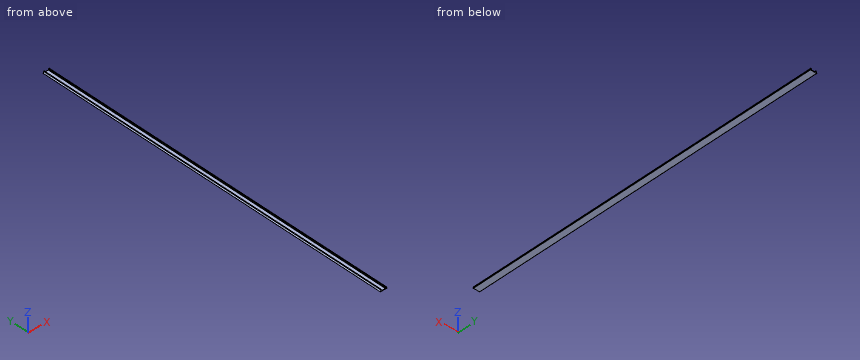
```python
from build123d import *

# Parameters (mm, degrees)
PROFILE_EXTRUDE_DEPTH = 500


with BuildPart() as part:
    # Profile Sketch → Profile Extrude (new body)
    with BuildSketch(Plane(origin=(0, 0, 0), x_dir=(1, 0, 0), z_dir=(0, 1, 0))):
        with BuildLine():
            Line((0, 0.762), (4.235793346, 0.762))
            ThreePointArc((4.235793346, 0.762), (4.559082566, 0.62808922), (4.692993346, 0.3048))
            ThreePointArc((4.692993346, 0.3048), (3.844388962, -0.212390939), (3.748927066, -1.20158399))
            ThreePointArc((3.748927066, -1.20158399), (3.415292673, -1.798270502), (2.889593346, -1.36125))
            Line((2.889593346, -1.36125), (2.889593346, -0.4572))
            ThreePointArc((2.889593346, -0.4572), (2.755682566, -0.13391078), (2.432393346, 0))
            Line((2.432393346, 0), (0, 0))
            Line((0, 0), (0, 0.762))
        make_face()
    profile_extrude = extrude(amount=PROFILE_EXTRUDE_DEPTH)

    # Profile Mirror: Profile Extrude across plane
    add(profile_extrude.mirror(Plane(origin=(0, 0, 0), x_dir=(0, 0, 1), z_dir=(1, 0, 0))))


solid = part.part
```
Source: CAD feature listing. Evaluate the final solid. Frame: model axes, mm. Give positions to 0.01 mm unless a question says otherwise; leave off trailing zeros. Order: outer loops, then holes, each group sorted by start corner. A loop starts at its lowest first (then second) coordinate and runs counter-clockwise, first axis right, second up. Notation, with made-up numbers: (35.25, 86) -> (40.25, 86) arc R20 cw to (40.25, 99) -> close; hole circle Ø6 at (20.25, -4). An arc over 180 degrees is marked (long way). Use a Markdown table: item, result.
Q1. First-contact query: P1, Ø0.7, axis at y = 144.5, z = 1, coming from the -X side; P2, Ø0.7, axis at y = 290, z = 0.5, coming from the +X side. Flat tips, straight axial feed; report the tip coordinate or a pass-through.
A:
| item | result |
|---|---|
| P1 | x = -3.78 |
| P2 | x = 3.89 |
Q2. Section B-B (x = -1). Return the cut outline in (y, z), and give its area (3 significant figures).
A:
| item | result |
|---|---|
| outline | (0, -0.76) -> (500, -0.76) -> (500, 0) -> (0, 0) -> close |
| area | 381 mm^2 |
Q3. Material intervals for line 1 (X direction, y = 278, z = 0.9); line 2 (X direction, y = 213, z = 1.5); line 3 (X direction, y = 121, z = -0.4), sorted ascending. Write a range as [from, to].
A:
| item | result |
|---|---|
| line 1 | [-3.68, -2.89], [2.89, 3.68] |
| line 2 | [-3.76, -2.91], [2.91, 3.76] |
| line 3 | [-4.68, 4.68] |
Q4. Section A-A (y = 308). Return the cut outline in (x, z), and give its area (3 significant figures).
A:
| item | result |
|---|---|
| outline | (-4.69, -0.3) arc R0.46 ccw to (-4.24, -0.76) -> (4.24, -0.76) arc R0.46 ccw to (4.69, -0.3) arc R1.11 cw to (3.75, 1.2) arc R0.44 ccw (long way) to (2.89, 1.36) -> (2.89, 0.46) arc R0.46 cw to (2.43, 0) -> (-2.43, 0) arc R0.46 cw to (-2.89, 0.46) -> (-2.89, 1.36) arc R0.44 ccw (long way) to (-3.75, 1.2) arc R1.11 cw to start |
| area | 9.86 mm^2 |
